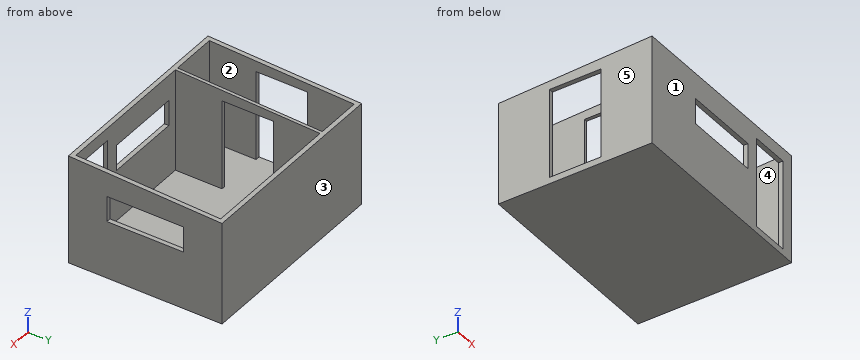
```python
from build123d import *

# Parameters (mm, degrees)
F0_W      = 101.6
F0_H      = 76.2
F1_DEPTH  = 3.175
F2_W      = 101.6
F2_H      = 76.2
F2_W_2    = 97.155
F2_H_2    = 71.755
F3_DEPTH  = 50.8
F4_W      = 1.5875
F4_H      = 71.755
F5_DEPTH  = 50.8
F6_W      = 19.05
F6_H      = 44.45
F6_W_2    = 38.1
F6_H_2    = 12.7
F7_DEPTH  = 25.4
F8_W      = 38.1
F8_H      = 12.7
F9_DEPTH  = 25.4
F11_DEPTH = 101.6
F12_W     = 25.4
F12_H     = 44.45
F13_DEPTH = 76.2


with BuildPart() as f1:
    # F0 (on Top) → F1 (new body)
    with BuildSketch(Plane.XY):
        Rectangle(F0_W, F0_H)
    extrude(amount=F1_DEPTH)

    # F2 (on face) → F3 (join)
    with BuildSketch(Plane.XY.offset(3.175)):
        Rectangle(F2_W, F2_H)
        Rectangle(F2_W_2, F2_H_2, mode=Mode.SUBTRACT)
    extrude(amount=F3_DEPTH)

    # F4 (on face) → F5 (join)
    with BuildSketch(Plane.XY.offset(3.175)):
        with Locations((-24.60625, 0)):
            Rectangle(F4_W, F4_H)
    extrude(amount=F5_DEPTH)

    # F6 (on face) → F7 (cut)
    with BuildSketch(Plane.XZ.offset(38.1)):
        with Locations((34.925, 25.4)):
            Rectangle(F6_W, F6_H)
        with Locations((0, 34.925)):
            Rectangle(F6_W_2, F6_H_2)
    extrude(amount=-F7_DEPTH, mode=Mode.SUBTRACT)

    # F8 (on face) → F9 (cut)
    with BuildSketch(Plane.YZ.offset(50.8)):
        with Locations((0, 34.925)):
            Rectangle(F8_W, F8_H)
    extrude(amount=-F9_DEPTH, mode=Mode.SUBTRACT)

    # F10 (on face) → F11 (cut, through all)
    with BuildSketch(Plane.YZ.offset(50.8)):
        Polygon((38.1, 53.975), (-38.1, 53.975), (38.1, 50.8), align=None)
    extrude(amount=-F11_DEPTH, mode=Mode.SUBTRACT)

    # F12 (on face) → F13 (cut)
    with BuildSketch(Plane(origin=(-50.8, 0, 0), x_dir=(0, -1, 0), z_dir=(-1, 0, 0))):
        with Locations((0, 25.4)):
            Rectangle(F12_W, F12_H)
    extrude(amount=-F13_DEPTH, mode=Mode.SUBTRACT)


solid = f1.part
```
Design review of the part built by this model. Coordinates are the model's own, in mm. Face numbers are marked on the shaded views. A direction names the side the tool comes from. Coordinates: 2 decimals unless noted, no trailing zeros. Loops run counter-clockwise (first coordinate to the right, second up) from the corner with the lowest first, then second, coordinate; pieces in that order, holes last. Notation, with made-up numbers: (60, 44) - (101, 44) arc R19 ccw to (101, 72) - close; hole circle Ø9 at (76.5, -25). An arc over 180 degrees is marked (long way). Use CSV: the item, a comma, the result in double quotes. Start each with the question number.
1) Tool access review of the marked faces 4 and 5: name each direction out of +Z, -Z, +X, -X, +Y, -Y from which nothing blocks a thin tool from reaching the whole face with its end or side.
2) Consider section D-D on y = 4. Write out the cut boundary in (x, z) (1 decimal), then the cut area to 3 significant figures.
3) Consider section A-A on x = 40.5. Write out the cut boundary in (y, z) (1 decimal).
4) For pin 1 Ø0.7 at (x, y) = (49.5, 2.5) entering from +Z; pin 2 Ø6 at (y, z) = (-3, 43) entering from -X; pin 3 Ø5 at (x, y) = (-28.5, 6) entering from +Z (3 decimals), all flat-tipped, find the tip position at first contact; note any pin that passes through.
5) Wall thickness on L1, parallel to X at y = 17, z = 8.5; L2, parallel to Y at x = -34, z = 45; L3, parallel to Z at x = -46, y = 23.5 (3 decimals): over which ranges is each line inside the solid? List them lowest first. Write a range as from..to.
6) The part is to be moulded in two halves that separate along Y. For the marked faces 1, 2 and 3, say which applies: +Y half, -Y half, draft (parallel to the pull), parting line (faces both ways), or undercut.
7) Consider section C-C on z = 23. Write out the cut boundary in (x, y).
8) Consider section B-B on z = 33.5. Give the number of separate pieces and of enclosed holes in the cut face, then the cut area to 3 significant figures.
Geometry says:
1,face 4,"+Z"
1,face 5,"+Z, -Z, -X, +Y, -Y"
2,outline,"(-50.8, 0) - (50.8, 0) - (50.8, 28.6) - (48.6, 28.6) - (48.6, 3.2) - (-50.8, 3.2) - close; (-50.8, 47.6) - (-48.6, 47.6) - (-48.6, 52.2) - (-50.8, 52.2) - close; (-25.4, 47.6) - (-23.8, 47.6) - (-23.8, 52.2) - (-25.4, 52.2) - close; (48.6, 41.3) - (50.8, 41.3) - (50.8, 52.2) - (48.6, 52.2) - close"
2,area,"421 mm^2"
3,outline,"(-38.1, 0) - (38.1, 0) - (38.1, 50.8) - (35.9, 50.9) - (35.9, 3.2) - (-38.1, 3.2) - close; (-38.1, 47.6) - (-35.9, 47.6) - (-35.9, 53.9) - (-38.1, 54) - close"
4,pin 1,"z = 52.3"
4,pin 2,"x = 48.58"
4,pin 3,"z = 3.175"
5,L1,"-50.8..-48.58, -25.4..-23.81, 48.58..50.8"
5,L2,"-38.1..-35.88, 35.88..38.1"
5,L3,"0..3.175"
6,face 1,"-Y half"
6,face 2,"undercut"
6,face 3,"+Y half"
7,outline,"(-50.8, -38.1) - (25.4, -38.1) - (25.4, -35.88) - (-23.81, -35.88) - (-23.81, -12.7) - (-25.4, -12.7) - (-25.4, -35.88) - (-48.58, -35.88) - (-48.58, -12.7) - (-50.8, -12.7) - close; (-50.8, 12.7) - (-48.58, 12.7) - (-48.58, 35.88) - (-25.4, 35.88) - (-25.4, 12.7) - (-23.81, 12.7) - (-23.81, 35.88) - (48.58, 35.88) - (48.58, -35.88) - (44.45, -35.88) - (44.45, -38.1) - (50.8, -38.1) - (50.8, 38.1) - (-50.8, 38.1) - close"
8,separate pieces,"4"
8,enclosed holes,"0"
8,area,"576 mm^2"
